Can you work these out from the drawing? Everything is in mm from the part's minimum corner. A direction names the side the tool comes from. Give positions to 0.01 mm unless a question says otherwise; leave off trailing zeros. Loops run counter-clockwise (first coordinate to the right, second up) from the corner with the lowest first, then second, coordinate; pieces in that order, holes last.
Q1. If we section it at B-B (z = 15): Please give me the cut outline in (x, y), plus the area to 3 significant figures.
Q2. For the marked faces 4, 5 and 6, which set-ups out of +Z, -Z, +X, -X, +Y, -Y let a thin tool reach every point of the face, with its end or its side?
Q3. We'd pull the mould along X, two halves only. Please class the marked faces 1, 2 and 3: +X half, -X half, draft (parallel to the pull), parting line (faces both ways), or undercut.
Q4. If we section it at C-C (y = 5.5): Please give me the cut outline in (x, z).
Q5. If we section it at D-D (z = 8.75): Please give me the cut outline in (x, y).
Q6. I need wall thicknesses on line 1 (Z direction, x = 4.5, y = 8.75); line 2 (Z direction, x = 5, y = 1.7); line 3 (X direction, y = 2.4, z = 15). Which ranges of each line are inside material? Lowest first, please.
Q7. Will these pins go through, and if not, where does the flat tip stop? P1, Ø2.5, axis at y = 9.5, z = 6, coming from the -X side; P2, Ø2, axis at x = 4, y = 5.5, coming from the -Z side; P3, Ø5, axis at x = 5, y = 8, coming from the -Z side; P4, Ø4, axis at y = 9, z = 8.5, coming from the +X side.
Q8. If we section it at A-A (x = 5): Please give me the cut outline in (y, z), plus the area to 3 significant figures.
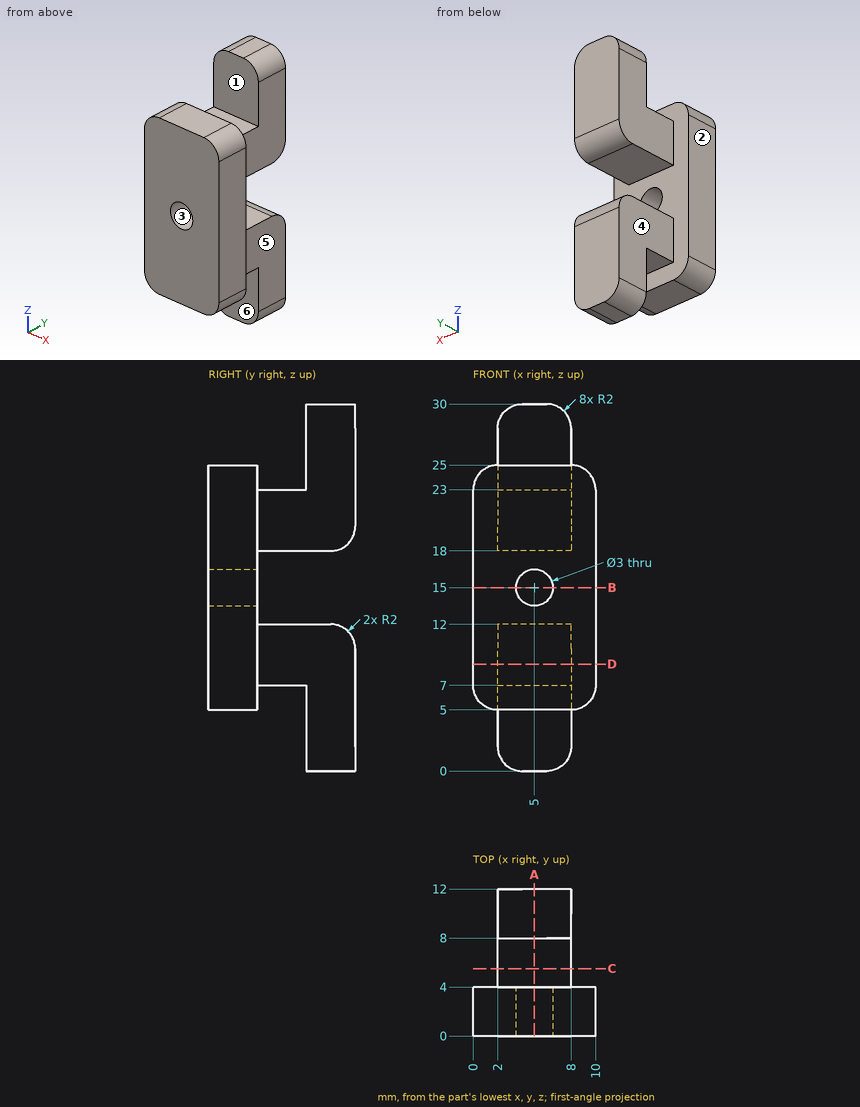
Check sheet entries:
1. outline: (0, 0) - (3.5, 0) - (3.5, 4) - (0, 4) - close; (6.5, 0) - (10, 0) - (10, 4) - (6.5, 4) - close
1. area: 28.0 mm2
2. face 4: +Z, -Z, -X, +Y
2. face 5: +Z, -Z, +X, +Y
2. face 6: -Z, +X, -X
3. face 1: draft
3. face 2: -X half
3. face 3: undercut
4. outline: (2, 7) - (8, 7) - (8, 12) - (2, 12) - close; (2, 18) - (8, 18) - (8, 23) - (2, 23) - close
5. outline: (0, 0) - (10, 0) - (10, 4) - (8, 4) - (8, 12) - (2, 12) - (2, 4) - (0, 4) - close
6. line 1: z = 0 to 12, 18 to 30
6. line 2: z = 5 to 13.5, 16.5 to 25
6. line 3: x = 0 to 3.5, 6.5 to 10
7. P1: stops at x = 2
7. P2: stops at z = 7
7. P3: stops at z = 0
7. P4: stops at x = 8
8. outline: (0, 5) - (4, 5) - (4, 7) - (8, 7) - (8, 0) - (12, 0) - (12, 10) arc R2 ccw to (10, 12) - (4, 12) - (4, 13.5) - (0, 13.5) - close; (0, 16.5) - (4, 16.5) - (4, 18) - (10, 18) arc R2 ccw to (12, 20) - (12, 30) - (8, 30) - (8, 23) - (4, 23) - (4, 25) - (0, 25) - close
8. area: 202 mm2
